Geometry check sheet. Reference: drawing and pictorial views, mm from the part's lowest x, y, z. A direction names the side the tool comes from. Coordinates: 2 decimals unless noted, no trailing zeros. Loops run counter-clockwise (first coordinate to the right, second up) from the corner with the lowest first, then second, coordinate; pieces in that order, holes last. Notation, with made-up numbers: (25, 48) - (62, 48) arc R4 ccw to (62, 54) - close; hole circle Ø8 at (-29, 29). An arc over 180 degrees is marked (long way). One line per item, written item: value.
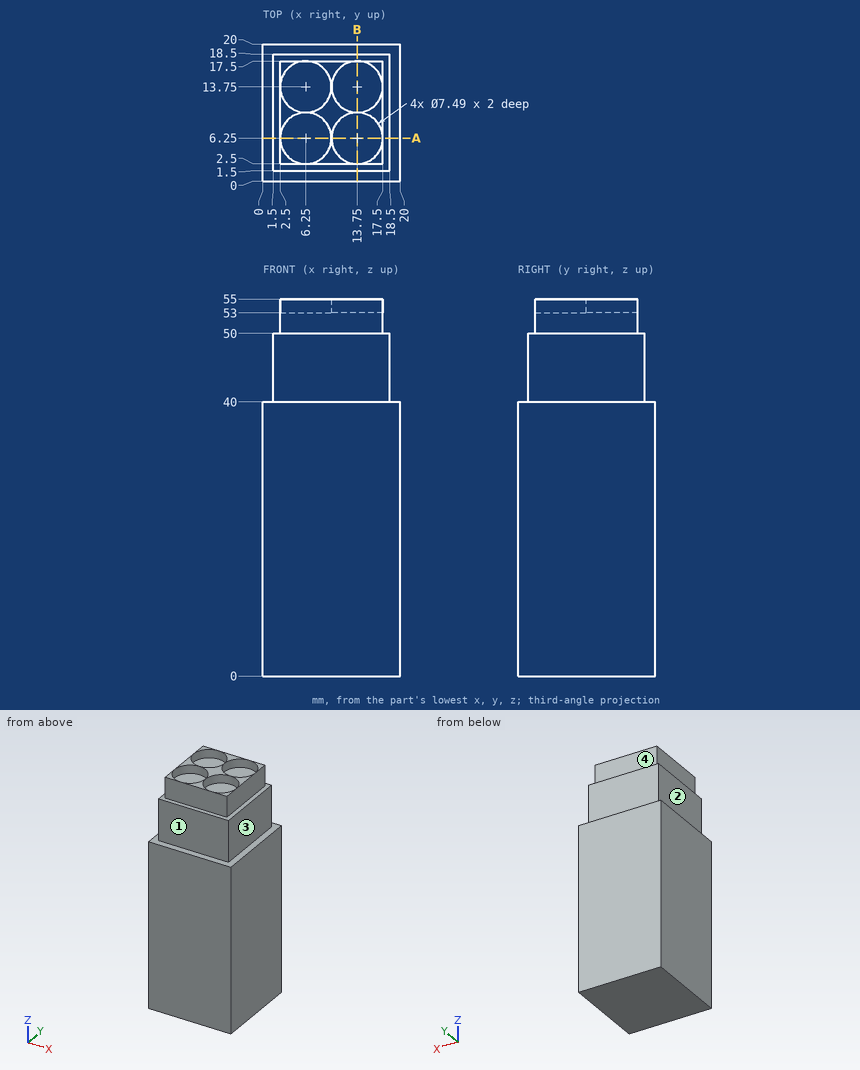
(1) Cross-section at A-A on y = 6.25. Record the cut outline in (x, z) (3 decimals).
Reply:
outline: (0, 0) - (20, 0) - (20, 40) - (18.5, 40) - (18.5, 50) - (17.5, 50) - (17.5, 55) - (17.495, 55) - (17.495, 53) - (10.005, 53) - (10.005, 55) - (9.995, 55) - (9.995, 53) - (2.505, 53) - (2.505, 55) - (2.5, 55) - (2.5, 50) - (1.5, 50) - (1.5, 40) - (0, 40) - close
(2) Go/stop test with flat-tipped pins: pin 1 Ø4 at (x, z) = (11, 52.5) entering from +Y; pin 2 Ø9.5 at (x, y) = (6.25, 6.25) entering from +Z; pin 3 Ø8 at (x, z) = (8.5, 47) entering from -Y; pin 4 Ø3 at (x, z) = (13.5, 43) entering from +Y. Record where each tip stops, or that it passes through.
Reply:
pin 1: y = 17.5
pin 2: z = 55
pin 3: y = 1.5
pin 4: y = 18.5
(3) Access from +Z, -Z, +X, -X, +Y, -Y to the whole of each face (thin tool, end or side, straight path). Record for the marked faces 1, 2, 3 and 4.
Reply:
face 1: +Z, +X, -X, -Y
face 2: +Z, -X, +Y, -Y
face 3: +Z, +X, +Y, -Y
face 4: +Z, +X, -X, +Y
(4) Material ranges on probe 1 along Z at (x, y) = (7.25, 6); probe 2 along Y at (x, z) = (2.5, 43.5); probe 3 along Z at (x, y) = (4.5, 1.75), recorded low to high. Write a range as from..to.
Reply:
probe 1: 0..53
probe 2: 1.5..18.5
probe 3: 0..50
